from build123d import *

# Parameters (mm, degrees)
SKETCH_1_W               = 12.5
SKETCH_1_H               = 30
EXTRUDE_1_DEPTH          = 10
CUT_EXTRUDE_1_DEPTH      = 20.080421903
CUT_EXTRUDE_1_DEPTH_BACK = 20.080421903
SKETCH_2_R               = 2.5
FILLET_1_R               = 2
CHAMFER_1_SIZE           = 2


with BuildPart() as part:
    # 草图1 → 凸台-拉伸1 (new body)
    with BuildSketch(Plane(origin=(0, 0, 0), x_dir=(0, 0, -1), z_dir=(1, 0, 0))):
        Rectangle(SKETCH_1_W, SKETCH_1_H)
    extrude(amount=EXTRUDE_1_DEPTH)

    # 草图2 → 切除-拉伸1 (cut, two sides: drawn at the far end of the back side and taken through both)
    with BuildSketch(Plane(origin=(10, 0, 0), x_dir=(0, 0, -1), z_dir=(1, 0, 0)).offset(-CUT_EXTRUDE_1_DEPTH_BACK)):
        with Locations((0, -10)):
            Circle(SKETCH_2_R)
    extrude(amount=CUT_EXTRUDE_1_DEPTH + CUT_EXTRUDE_1_DEPTH_BACK, mode=Mode.SUBTRACT)

    # 圆角1
    fillet_1_edges = [part.edges().sort_by_distance(p)[0] for p in [
        (5, -15, -6.25),
        (5, -15, 6.25),
    ]]
    fillet(fillet_1_edges, radius=FILLET_1_R)

    # 倒角1
    chamfer_1_edges = [part.edges().sort_by_distance(p)[0] for p in [
        (0, 15, 0),
    ]]
    chamfer(chamfer_1_edges, length=CHAMFER_1_SIZE)


solid = part.part
Can you work these out from the model? Positions are in its coordinate system, mm. Give positions to 0.01 mm unless a question says otherwise; leave off trailing zeros. Loops run counter-clockwise (first coordinate to the right, second up) from the corner with the lowest first, then second, coordinate; pieces in that order, holes last. Notation, with made-up numbers: (49.25, 9) - (106.25, 9) arc R6 cw to (106.25, 20) - close; hole circle Ø10 at (-25, 57.25). An arc over 180 degrees is marked (long way). One line per item, written item: value.
(1) I need wall thicknesses on line 1 along Z through (x, y) = (3, -10); line 2 along Y through (x, z) = (5.25, 0); line 3 along Y through (x, z) = (7, -0.5). Which ranges of each line are inside material? Lowest first, please.
Verdict:
line 1: -6.25 to -2.5, 2.5 to 6.25
line 2: -15 to -12.5, -7.5 to 15
line 3: -15 to -12.45, -7.55 to 15
(2) I'm going to push a flat-ended pin straight in: pin 1 (6.5 mm diameter, centred on y = -10, z = 0, fed in from -X). Where does the tip first touch, or does it pass through?
Verdict:
pin 1: x = 0
(3) If we section it at C-C, the plane x = 9.5: List the corners of the cut face in (y, z) for me, plus the area to 3 significant figures.
Verdict:
outline: (-15, -4.25) arc R2 ccw to (-13, -6.25) - (15, -6.25) - (15, 6.25) - (-13, 6.25) arc R2 ccw to (-15, 4.25) - close; hole circle Ø5 at (-10, 0)
area: 354 mm^2
(4) If we section it at A-A, the plane z = 0: List the corners of the cut face in (x, y) for me.
Verdict:
outline: (0, -15) - (10, -15) - (10, -12.5) - (0, -12.5) - close; (0, -7.5) - (10, -7.5) - (10, 15) - (2, 15) - (0, 13) - close
(5) If we section it at D-D, the plane z = 1.25: List the corners of the cut face in (x, y) for me, plus the area to 3 significant figures.
Verdict:
outline: (0, -15) - (10, -15) - (10, -12.17) - (0, -12.17) - close; (0, -7.83) - (10, -7.83) - (10, 15) - (2, 15) - (0, 13) - close
area: 255 mm^2
(6) If we mould it in two halves opening along Z, with no side actions, what happens to faces 1 (the face through (4.93, -12.44, 0.54)), 2 (the face through (5, -15, 0)), 3 (the face through (5.07, -14.4, 5.68)), 4 (the face through (5.07, -14.43, -5.65))? For each: released by +Z, released by -Z, zero draft, split by the parting line, or undercut.
Verdict:
face 1: undercut
face 2: zero draft
face 3: released by +Z
face 4: released by -Z
(7) If we section it at B-B, the plane y = -10: List the corners of the cut face in (x, z) for me.
Verdict:
outline: (0, -6.25) - (10, -6.25) - (10, -2.5) - (0, -2.5) - close; (0, 2.5) - (10, 2.5) - (10, 6.25) - (0, 6.25) - close
